```python
from build123d import *

# Parameters (mm, degrees)
F0_R     = 2.1
F1_DEPTH = 310


with BuildPart() as f1:
    # F0 (on Front) → F1 (new body)
    with BuildSketch(Plane.XZ):
        with BuildLine():
            ThreePointArc((9.944745, 8.840758), (9.651851, 9.547865), (8.944745, 9.840758))
            Line((8.944745, 9.840758), (2.944745, 9.840758))
            Line((2.944745, 9.840758), (2.944745, 7.840758))
            Line((2.944745, 7.840758), (6.884085, 7.840758))
            Line((6.884085, 7.840758), (2.884085, 3.840758))
            Line((2.884085, 3.840758), (-2.994595, 3.840758))
            Line((-2.994595, 3.840758), (-6.994595, 7.840758))
            Line((-6.994595, 7.840758), (-3.055255, 7.840758))
            Line((-3.055255, 7.840758), (-3.055255, 9.840758))
            Line((-3.055255, 9.840758), (-9.055255, 9.840758))
            ThreePointArc((-9.055255, 9.840758), (-9.762362, 9.547865), (-10.055255, 8.840758))
            Line((-10.055255, 8.840758), (-10.055255, 2.840758))
            Line((-10.055255, 2.840758), (-8.055255, 2.840758))
            Line((-8.055255, 2.840758), (-8.055255, 6.780098))
            Line((-8.055255, 6.780098), (-4.055255, 2.780098))
            Line((-4.055255, 2.780098), (-4.055255, -3.098581))
            Line((-4.055255, -3.098581), (-8.055255, -7.098581))
            Line((-8.055255, -7.098581), (-8.055255, -3.159242))
            Line((-8.055255, -3.159242), (-10.055255, -3.159242))
            Line((-10.055255, -3.159242), (-10.055255, -9.159242))
            ThreePointArc((-10.055255, -9.159242), (-9.762362, -9.866348), (-9.055255, -10.159242))
            Line((-9.055255, -10.159242), (-3.055255, -10.159242))
            Line((-3.055255, -10.159242), (-3.055255, -8.159242))
            Line((-3.055255, -8.159242), (-6.994595, -8.159242))
            Line((-6.994595, -8.159242), (-2.994595, -4.159242))
            Line((-2.994595, -4.159242), (2.884085, -4.159242))
            Line((2.884085, -4.159242), (6.884085, -8.159242))
            Line((6.884085, -8.159242), (2.944745, -8.159242))
            Line((2.944745, -8.159242), (2.944745, -10.159242))
            Line((2.944745, -10.159242), (8.944745, -10.159242))
            ThreePointArc((8.944745, -10.159242), (9.651851, -9.866348), (9.944745, -9.159242))
            Line((9.944745, -9.159242), (9.944745, -3.159242))
            Line((9.944745, -3.159242), (7.944745, -3.159242))
            Line((7.944745, -3.159242), (7.944745, -7.098581))
            Line((7.944745, -7.098581), (3.944745, -3.098581))
            Line((3.944745, -3.098581), (3.944745, 2.780098))
            Line((3.944745, 2.780098), (7.944745, 6.780098))
            Line((7.944745, 6.780098), (7.944745, 2.840758))
            Line((7.944745, 2.840758), (9.944745, 2.840758))
            Line((9.944745, 2.840758), (9.944745, 8.840758))
        make_face()
        with Locations((-0.055255, -0.159242)):
            Circle(F0_R, mode=Mode.SUBTRACT)
    extrude(amount=F1_DEPTH)


solid = f1.part
```
The listing builds one solid part. Answer for the finished solid, in the listing's coordinates (mm). A direction names the side the tool comes from. Give positions to 0.01 mm unless a question says otherwise; leave off trailing zeros.
1) Consider line 1 along Z through (x, y) = (-0.25, -221.5); line 2 along Z through (x, y) = (3.5, -77); line 3 along X through (y, z) = (-73.5, 3). Determine where each line is inside the solid, lowest interval first.
Reported:
line 1: z = -4.16 to -2.25, 1.93 to 3.84
line 2: z = -10.16 to -8.16, -4.78 to 4.46, 7.84 to 9.84
line 3: x = -10.06 to -8.06, -4.28 to 4.16, 7.94 to 9.94
2) For faces 1 (the face through (0, -153, 3.841)), 2 (the face through (0, -153, -4.159)), 3 (the face through (9.945, -153, 6)), 4 (the face through (3.945, -153, 0)), determine the directions among +Z, -Z, +X, -X, +Y, -Y from which every point of the face is accessible in a straight line to the end or side of a thin tool.
Reported:
face 1: +Z, +Y, -Y
face 2: -Z, +Y, -Y
face 3: +Z, -Z, +X, +Y, -Y
face 4: +X, +Y, -Y
3) Determine the mould class of faces 5 (the face through (-0.2, -310, 2.2)), 6 (the face through (-6, -153, 9.841)), 7 (the face through (-4.055, -153, 0)), 8 (the face through (6, -153, -10.159)) for opening direction Z: pulls with the +Z half, pulls with the -Z half, needs draft (parallel to the pull), parting line crosses it, or undercut.
Reported:
face 5: needs draft
face 6: pulls with the +Z half
face 7: undercut
face 8: pulls with the -Z half
4) Given P1, Ø1.8, axis at x = -1.5, y = -217, coming from the +Z side; P2, Ø1, axis at x = 1, y = -80, coming from the -Z side; P3, Ø4.5, axis at y = -153, z = 0, coming from the -X side, each flat-ended and moving along its own axis, determine where each tip first touches the part or whether it passes through.
Reported:
P1: stops at z = 3.84
P2: stops at z = -4.16
P3: stops at x = -4.06
